Design review of the part shown in the three views and the two pictorial views. Dimensions are in mm from the part's minimum x, y and z. Coordinates: 2 decimals unless noted, no trailing zeros. Order: outer loops, then holes, each group sorted by start corner. A loop starts at its lowest first (then second) coordinate and runs counter-clockwise, first axis right, second up. Notation, with made-up numbers: M 84.5,29 L 119.5,29 A17 cw 119.5,35 Z; hole C -19,15 d7. An arc over 180 degrees is marked long. Use CSV: the item, a comma, the result in double quotes.
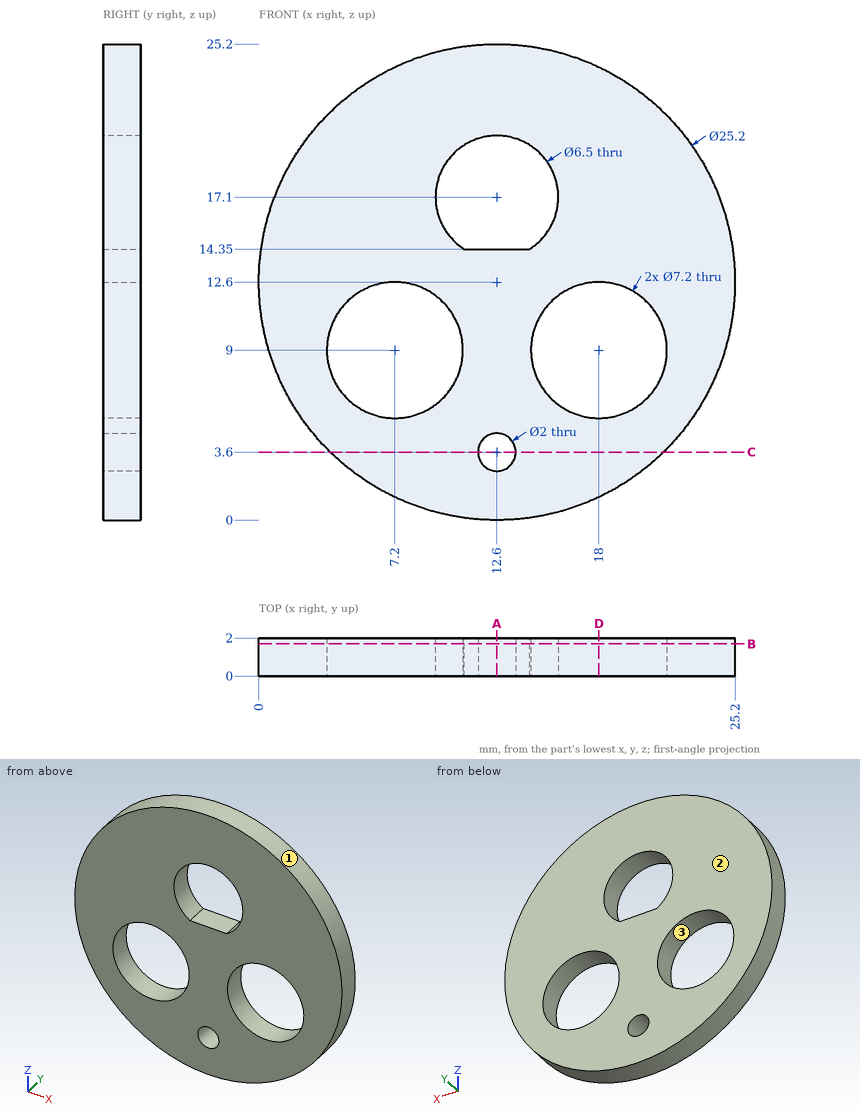
(1) Wall thickness on probe 1 along Z at (x, y) = (12.25, 1.1); probe 2 along X at (y, z) = (1.45, 9); probe 3 along Z at (x, y) = (7.2, 0.5): over which ranges is each line inside the solid? List them lowest first.
The answers:
probe 1,"z = 0 to 2.66, 4.54 to 14.35, 20.33 to 25.2"
probe 2,"x = 0.53 to 3.6, 10.8 to 14.4, 21.6 to 24.67"
probe 3,"z = 1.22 to 5.4, 12.6 to 23.98"
(2) Add section B-B on y = 1.7. State the section outline as (x, z) points, and give its area (3 significant figures).
The answers:
outline,"C 12.6,12.6 d25.2; hole C 7.2,9 d7.2; hole M 10.87,14.35 L 14.33,14.35 A3.25 ccw long Z; hole C 12.6,3.6 d2; hole C 18,9 d7.2"
area,"382 mm2"
(3) Add section C-C on z = 3.6. State the section outline as (x, y) points, and give its area (3 significant figures).
The answers:
outline,"M 3.78,0 L 11.6,0 L 11.6,2 L 3.78,2 Z; M 13.6,0 L 21.42,0 L 21.42,2 L 13.6,2 Z"
area,"31.3 mm2"
(4) Add section A-A on x = 12.6. State the section outline as (y, z) points.
The answers:
outline,"M 0,0 L 2,0 L 2,2.6 L 0,2.6 Z; M 0,4.6 L 2,4.6 L 2,14.35 L 0,14.35 Z; M 0,20.35 L 2,20.35 L 2,25.2 L 0,25.2 Z"
(5) Add section D-D on x = 18. State the section outline as (y, z) points, and give its area (3 significant figures).
The answers:
outline,"M 0,1.22 L 2,1.22 L 2,5.4 L 0,5.4 Z; M 0,12.6 L 2,12.6 L 2,23.98 L 0,23.98 Z"
area,"31.1 mm2"
(6) Clearance check with flat-ended pins moving along their axes: P1, Ø1, axis at y = 0.5, z = 8.5, coming from the +X side; P2, Ø4, axis at x = 16.5, z = 11.5, coming from the -Y side. State where each tip first meets the part, or that it passes through.
The answers:
P1,"stops at x = 24.67"
P2,"stops at y = 0"
(7) The part is to be moulded in two halves that separate along Z. For the marked faces 1, 2 and 3, say which applies: pulls with the +Z half, pulls with the -Z half, needs draft (parallel to the pull), parting line crosses it, or undercut.
The answers:
face 1,"parting line crosses it"
face 2,"needs draft"
face 3,"undercut"
